Input: part model. Units: mm. Frame: model coordinates. A direction names the side the tool comes from. Give positions to 0.01 mm unless a question says otherwise; leave off trailing zeros. Write each loop counter-clockwise with the first axis right and the second up, starting at its lowest first coordinate (ties: lowest second). Pieces come first, ordered by that corner, then holes. Notation, with made-up numbers: (86.25, -31.5) -> (137.25, -31.5) arc R20 cw to (137.25, 4.5) -> close; hole circle Ø7 at (74, -27.75). An arc over 180 degrees is marked (long way). Return JSON: item names as keys, results as strings. Group by question number.
Item 1: Section D-D, the plane x = 9.5. Return loops of the section in (y, z) (3 decimals).
Item 2: Section A-A, the plane y = 110.5. Return loops of the section in (x, z) (3 decimals).
Item 3: Mould query, pull axis X, two halves, no side actions, for faces 1 (the face through (6.35, 357, 21)), 2 (the face through (11, 0, 28)), 3 (the face through (15.875, 185, 97)), 4 (the face through (11, 189, 92.075)). Classes: released by +X, released by -X, zero draft, split by the parting line, or undercut.
Item 4: Section B-B, the plane z = 13.5. Return loops of the section in (x, y) (3 decimals), then the cut area to 3 significant figures.
Item 5: Line query: line 1 (X direction, y = 194, z = 93.5) (3 decimals); line 2 (X direction, y = 350.5, z = 24.5) (3 decimals); line 3 (Z direction, x = 11.75, y = 98) (3 decimals). Output: solid intervals per line, ascending. Write a range as [from, to].
Item 6: Set-up query: faces 5 (the face through (15.875, 357, 21)), 6 (the face through (11, 357, 41.275)), 7 (the face through (11, 188, 19.05)), 8 (the face through (6.35, 18, 28)), 9 (the face through (6.35, 189, 97)). Return all of +Z, -Z, +X, -X, +Y, -Y with unobstructed straight access to the full face (end or side cutting, diameter ignored); none if empty.
Item 7: Pin query (flat end, axial travel): P1, Ø2, axis at x = 18.5, z = 84.5, coming from the -Y side (3 decimals); P2, Ø11, axis at x = 14.5, y = 212, coming from the -Z side; P3, Ø7.5, axis at x = 10, y = 352.5, coming from the +Z side (3 decimals). Return the tip coordinate at first contact, or that it passes through.
Item 8: Section C-C, the plane z = 54. Return loops of the section in (x, y) (3 decimals).
from build123d import *

# Parameters (mm, degrees)
F0_W     = 374.65
F0_H     = 101.6
F1_DEPTH = 22.225
F2_W     = 9.525
F2_H     = 34.925
F2_H_2   = 304.8
F3_DEPTH = 9.525
F2_W_2   = 6.35
F4_DEPTH = 101.6
F5_W     = 34.925
F5_H     = 50.8
F6_DEPTH = 9.525
F8_DEPTH = 22.225
F9_DEPTH = 15.875


with BuildPart() as f1:
    # F0 (on Right) → F1 (new body)
    with BuildSketch(Plane.YZ):
        with Locations((187.325, 50.8)):
            Rectangle(F0_W, F0_H)
    extrude(amount=F1_DEPTH)

    # F2 (on face) → F3 (cut)
    with BuildSketch(Plane.XY.offset(101.6)):
        with Locations((11.1125, 357.1875)):
            Rectangle(F2_W, F2_H)
        with Locations((11.1125, 187.325)):
            Rectangle(F2_W, F2_H_2)
        with Locations((11.1125, 17.4625)):
            Rectangle(F2_W, F2_H)
    extrude(amount=-F3_DEPTH, mode=Mode.SUBTRACT)

    # F2 (on face) → F4 (cut, through all)
    with BuildSketch(Plane.XY.offset(101.6)):
        with Locations((19.05, 357.1875)):
            Rectangle(F2_W_2, F2_H)
        with Locations((3.175, 357.1875)):
            Rectangle(F2_W_2, F2_H)
        with Locations((3.175, 17.4625)):
            Rectangle(F2_W_2, F2_H)
        with Locations((19.05, 17.4625)):
            Rectangle(F2_W_2, F2_H)
    extrude(amount=-F4_DEPTH, mode=Mode.SUBTRACT)

    # F5 (on face) → F6 (cut, through all)
    with BuildSketch(Plane(origin=(6.35, 0, 0), x_dir=(0, -1, 0), z_dir=(-1, 0, 0))):
        with Locations((-357.1875, 66.675)):
            Rectangle(F5_W, F5_H)
        with Locations((-17.4625, 66.675)):
            Rectangle(F5_W, F5_H)
    extrude(amount=-F6_DEPTH, mode=Mode.SUBTRACT)

    # F7 (on Right) → F8 (cut, through all)
    with BuildSketch(Plane.YZ):
        Polygon((257.175, 0), (257.175, 19.05), (212.725, 19.05), (161.925, 19.05), (117.475, 19.05), (117.475, 0), align=None)
    extrude(amount=F8_DEPTH, mode=Mode.SUBTRACT)

    # F9 (add): a face of the model
    f9_faces = [f1.faces().sort_by_distance(p)[0] for p in [
        (11.1125, 17.4625, 41.275),
    ]]
    extrude(f9_faces, amount=F9_DEPTH)


solid = f1.part
Answer below:
{
 "1": {"outline": "(0, 0) -> (117.475, 0) -> (117.475, 19.05) -> (257.175, 19.05) -> (257.175, 0) -> (374.65, 0) -> (374.65, 41.275) -> (339.725, 41.275) -> (339.725, 92.075) -> (34.925, 92.075) -> (34.925, 57.15) -> (0, 57.15) -> close"},
 "2": {"outline": "(0, 0) -> (22.225, 0) -> (22.225, 101.6) -> (15.875, 101.6) -> (15.875, 92.075) -> (6.35, 92.075) -> (6.35, 101.6) -> (0, 101.6) -> close"},
 "3": {"face 1": "released by -X", "face 2": "zero draft", "face 3": "undercut", "face 4": "undercut"},
 "4": {"outline": "(0, 34.925) -> (6.35, 34.925) -> (6.35, 0) -> (15.875, 0) -> (15.875, 34.925) -> (22.225, 34.925) -> (22.225, 117.475) -> (0, 117.475) -> close; (0, 257.175) -> (22.225, 257.175) -> (22.225, 339.725) -> (15.875, 339.725) -> (15.875, 374.65) -> (6.35, 374.65) -> (6.35, 339.725) -> (0, 339.725) -> close", "area": "4,330 mm2"},
 "5": {"line 1": "x = [0, 6.35], [15.875, 22.225]", "line 2": "x = [6.35, 15.875]", "line 3": "z = [0, 92.075]"},
 "6": {"face 5": "+Z, -Z, +X, +Y", "face 6": "+Z, +X, -X, +Y", "face 7": "-Z, +X, -X", "face 8": "+Z, -Z, -X, -Y", "face 9": "+Z, +Y, -Y"},
 "7": {"P1": "stops at y = 34.925", "P2": "stops at z = 19.05", "P3": "stops at z = 41.275"},
 "8": {"outline": "(0, 34.925) -> (6.35, 34.925) -> (6.35, 0) -> (15.875, 0) -> (15.875, 34.925) -> (22.225, 34.925) -> (22.225, 339.725) -> (0, 339.725) -> close"}
}
